Geometry check sheet. Reference: drawing and pictorial views, mm from the part's lowest x, y, z. A direction names the side the tool comes from. Coordinates: 2 decimals unless noted, no trailing zeros. Loops run counter-clockwise (first coordinate to the right, second up) from the corner with the lowest first, then second, coordinate; pieces in that order, holes last.
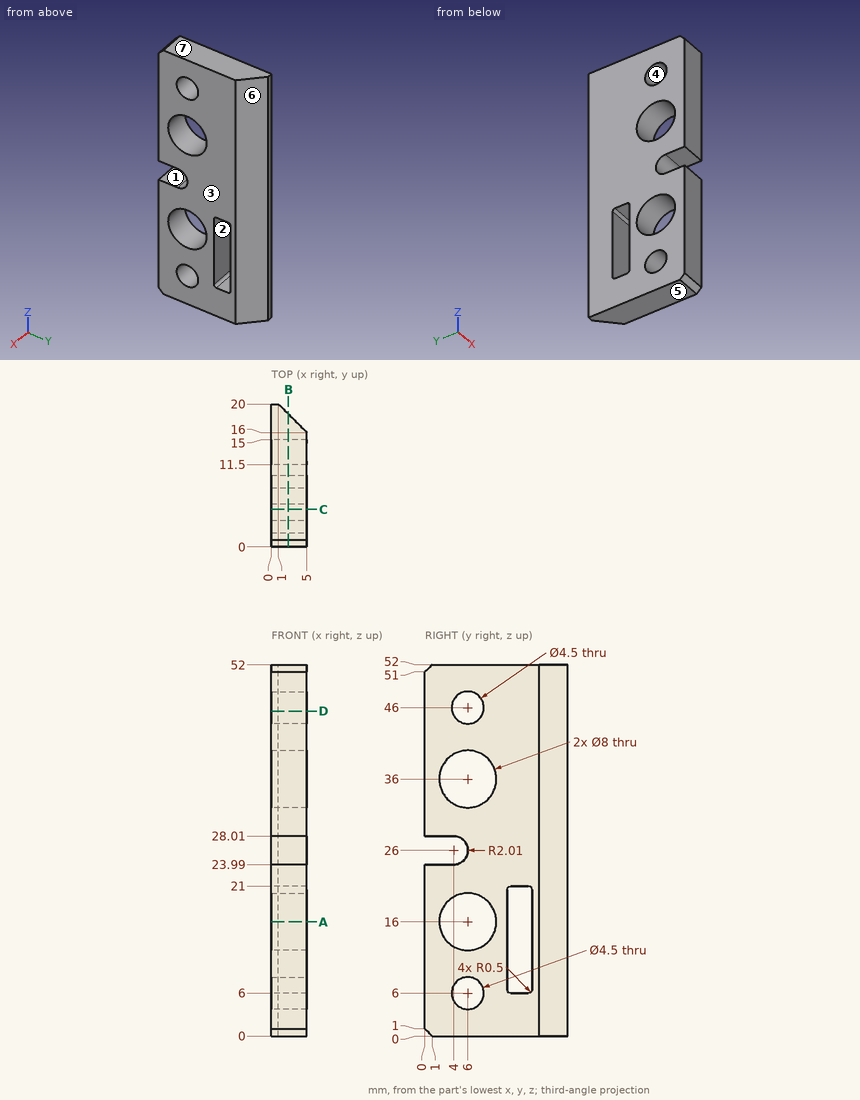
1) Material ranges on probe 1 along Z at (x, y) = (1.4, 7.75); probe 2 along Z at (x, y) = (1.15, 12); probe 3 along Y at (x, z) = (2.3, 14), recorded low to high.
Data:
probe 1: z = 0 to 4.59, 7.41 to 12.4, 19.6 to 32.4, 39.6 to 44.59, 47.41 to 52
probe 2: z = 0 to 6, 21 to 52
probe 3: y = 0 to 2.54, 9.46 to 11.5, 15 to 18.7
2) Section check C-C on y = 5.25. Record the cut outline in (x, z), and give its area (3 significant figures).
Data:
outline: (0, 0) - (5, 0) - (5, 3.88) - (0, 3.88) - close; (0, 8.12) - (5, 8.12) - (5, 12.07) - (0, 12.07) - close; (0, 19.93) - (5, 19.93) - (5, 24.43) - (0, 24.43) - close; (0, 27.57) - (5, 27.57) - (5, 32.07) - (0, 32.07) - close; (0, 39.93) - (5, 39.93) - (5, 43.88) - (0, 43.88) - close; (0, 48.12) - (5, 48.12) - (5, 52) - (0, 52) - close
area: 123 mm2
3) Section check B-B on x = 2.4. Record the cut outline in (y, z), and give its area (3 significant figures).
Data:
outline: (0, 1) - (1, 0) - (18.6, 0) - (18.6, 52) - (1, 52) - (0, 51) - (0, 28.01) - (4, 28.01) arc R2.01 cw to (4, 23.99) - (0, 23.99) - close; hole circle Ø8 at (6, 16); hole circle Ø8 at (6, 36); hole circle Ø4.5 at (6, 6); hole circle Ø4.5 at (6, 46); hole (11.5, 6.5) arc R0.5 ccw to (12, 6) - (14.5, 6) arc R0.5 ccw to (15, 6.5) - (15, 20.5) arc R0.5 ccw to (14.5, 21) - (12, 21) arc R0.5 ccw to (11.5, 20.5) - close
area: 759 mm2
4) Section check A-A on z = 16. Record the cut outline in (x, y).
Data:
outline: (0, 0) - (5, 0) - (5, 2) - (0, 2) - close; (0, 10) - (5, 10) - (5, 11.5) - (0, 11.5) - close; (0, 15) - (5, 15) - (5, 16) - (1, 20) - (0, 20) - close
5) Section check D-D on z = 45.5. Record the cut outline in (x, y).
Data:
outline: (0, 0) - (5, 0) - (5, 3.81) - (0, 3.81) - close; (0, 8.19) - (5, 8.19) - (5, 16) - (1, 20) - (0, 20) - close
6) Access from +Z, -Z, +X, -X, +Y, -Y to the whole of each face (thin tool, end or side, straight path). Record for the marked faces 1, 2 and 3.
Data:
face 1: +X, -X, -Y
face 2: +X, -X
face 3: +Z, -Z, +X, +Y, -Y
7) Mould release check, pull along Z, two halves, no side actions. Record for the marked faces 4, 5, 6 and 7: +Z half, -Z half, draft (parallel to the pull), parting line (faces both ways), or undercut.
Data:
face 4: undercut
face 5: -Z half
face 6: draft
face 7: +Z half
